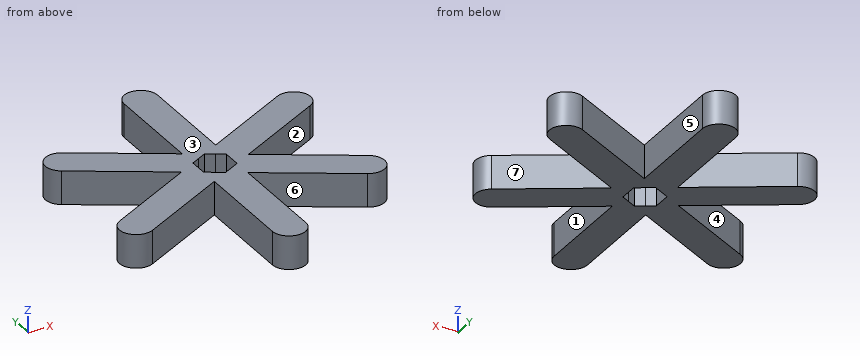
from build123d import *

# Parameters (mm, degrees)
F1_DEPTH = 12.7


with BuildPart() as f1:
    # F0 (on Top) → F1 (new body)
    with BuildSketch(Plane.XY):
        Polygon((-6.35, -3.6661742094), (-6.35, 0), (-6.35, 3.6661742094), (-12.7, 0), align=None)
        Polygon((0, -7.3323484187), (-3.175, -5.499261314), (-6.35, -3.6661742094), (-6.35, -10.9985226281), align=None)
        Polygon((6.35, 3.6661742094), (6.35, 0), (6.35, -3.6661742094), (12.7, 0), align=None)
        with BuildLine():
            Line((-12.7, 0), (-6.35, 3.6661742094))
            Line((-6.35, 3.6661742094), (-6.35, 10.9985226281))
            Line((-6.35, 10.9985226281), (-40.8190905122, 30.899261314))
            ThreePointArc((-40.8190905122, 30.899261314), (-49.4933518263, 28.575), (-47.1690905122, 19.900738686))
            Line((-47.1690905122, 19.900738686), (-12.7, 0))
        make_face()
        Polygon((-6.35, 10.9985226281), (-6.35, 3.6661742094), (-3.175, 5.499261314), (0, 7.3323484187), align=None)
        with BuildLine():
            Line((-6.35, -10.9985226281), (-6.35, -3.6661742094))
            Line((-6.35, -3.6661742094), (-12.7, 0))
            Line((-12.7, 0), (-47.1690905122, -19.900738686))
            ThreePointArc((-47.1690905122, -19.900738686), (-49.4933518263, -28.575), (-40.8190905122, -30.899261314))
            Line((-40.8190905122, -30.899261314), (-6.35, -10.9985226281))
        make_face()
        Polygon((6.35, -3.6661742094), (3.175, -5.499261314), (0, -7.3323484187), (6.35, -10.9985226281), align=None)
        with BuildLine():
            Line((6.35, -10.9985226281), (0, -7.3323484187))
            Line((0, -7.3323484187), (-6.35, -10.9985226281))
            Line((-6.35, -10.9985226281), (-6.35, -50.8))
            ThreePointArc((-6.35, -50.8), (0, -57.15), (6.35, -50.8))
            Line((6.35, -50.8), (6.35, -10.9985226281))
        make_face()
        Polygon((3.175, 5.499261314), (6.35, 3.6661742094), (6.35, 10.9985226281), (0, 7.3323484187), align=None)
        with BuildLine():
            Line((6.35, 10.9985226281), (6.35, 3.6661742094))
            Line((6.35, 3.6661742094), (12.7, 0))
            Line((12.7, 0), (47.1690905122, 19.900738686))
            ThreePointArc((47.1690905122, 19.900738686), (49.4933518263, 28.575), (40.8190905122, 30.899261314))
            Line((40.8190905122, 30.899261314), (6.35, 10.9985226281))
        make_face()
        with BuildLine():
            Line((12.7, 0), (6.35, -3.6661742094))
            Line((6.35, -3.6661742094), (6.35, -10.9985226281))
            Line((6.35, -10.9985226281), (40.8190905122, -30.899261314))
            ThreePointArc((40.8190905122, -30.899261314), (49.4933518263, -28.575), (47.1690905122, -19.900738686))
            Line((47.1690905122, -19.900738686), (12.7, 0))
        make_face()
        with BuildLine():
            Line((-6.35, 50.8), (-6.35, 10.9985226281))
            Line((-6.35, 10.9985226281), (0, 7.3323484187))
            Line((0, 7.3323484187), (6.35, 10.9985226281))
            Line((6.35, 10.9985226281), (6.35, 50.8))
            ThreePointArc((6.35, 50.8), (0, 57.15), (-6.35, 50.8))
        make_face()
    extrude(amount=-F1_DEPTH)


solid = f1.part
Could you check a few things on this model? Use its own coordinates, in mm. Face numbers are marked on the shaded views. A direction names the side the tool comes from. Round coordinates to 2 decimals unless told otherwise and drop trailing zeros. Loops run counter-clockwise (first coordinate to the right, second up) from the corner with the lowest first, then second, coordinate; pieces in that order, holes last. Notation, with made-up numbers: (78, 68.5) - (111, 68.5) arc R29 cw to (111, 102.5) - close; hole circle Ø5 at (-11, 50.5). An arc over 180 degrees is marked (long way). Write item = value, one per line.
1) Imagine slicing it at B-B (z = -2.5). Please give me the cut outline in (x, y) (3 decimals).
Computed:
outline = (-47.169, -19.901) arc R6.35 ccw to (-40.819, -30.899) - (-6.35, -10.999) - (-6.35, -50.8) arc R6.35 ccw to (6.35, -50.8) - (6.35, -10.999) - (40.819, -30.899) arc R6.35 ccw to (47.169, -19.901) - (12.7, 0) - (47.169, 19.901) arc R6.35 ccw to (40.819, 30.899) - (6.35, 10.999) - (6.35, 50.8) arc R6.35 ccw to (-6.35, 50.8) - (-6.35, 10.999) - (-40.819, 30.899) arc R6.35 ccw to (-47.169, 19.901) - (-12.7, 0) - close; hole (-6.35, -3.666) - (0, -7.332) - (6.35, -3.666) - (6.35, 3.666) - (0, 7.332) - (-6.35, 3.666) - close
2) If we mould it in two halves opening along X, with no side actions, what happens to the marked faces 1, 2 and 3? For each: pulls with the +X half, pulls with the -X half, needs draft (parallel to the pull), parting line crosses it, or undercut.
Computed:
face_1 = undercut
face_2 = pulls with the +X half
face_3 = needs draft
3) On a 3-axis mill with a long thin cutter (end or side, diameter ignored), from which of +Z, -Z, +X, -X, +Y, -Y can I reach the whole of each face in a straight line? I mean the marked faces 4, 5, 6 and 7. Say none if no direction works.
Computed:
face_4 = +Z, -Z, -X
face_5 = +Z, -Z, +Y
face_6 = +Z, -Z, -Y
face_7 = +Z, -Z, +X
4) Imagine slicing it at C-C (y = -13). Please give me the cut outline in (x, z), and give its area (3 significant figures).
Computed:
outline = (-35.22, -12.7) - (-9.82, -12.7) - (-9.82, 0) - (-35.22, 0) - close; (-6.35, -12.7) - (6.35, -12.7) - (6.35, 0) - (-6.35, 0) - close; (9.82, -12.7) - (35.22, -12.7) - (35.22, 0) - (9.82, 0) - close
area = 806 mm2
5) I'm going to push flat-ended pins straight in: P1, Ø4, axis at y = 21, z = -3.5, coming from the +X side; P2, Ø2, axis at y = 0, z = -4, coming from the -X side. Where does each tip first touch, or does it pass through?
Computed:
P1 = 49.87
P2 = -14.43
6) Imagine slicing it at A-A (x = 14). Please give me the cut outline in (y, z), and give its area (3 significant figures).
Computed:
outline = (-15.42, -12.7) - (-0.75, -12.7) - (-0.75, 0) - (-15.42, 0) - close; (0.75, -12.7) - (15.42, -12.7) - (15.42, 0) - (0.75, 0) - close
area = 372 mm2
7) I need wall thicknesses on line 1 along X through (y, z) = (-25.5, -5.25); line 2 along X through (y, z) = (-29, -11.75) (3 decimals); line 3 along X through (y, z) = (-44, -1). Which ranges of each line are inside material? Lowest first, please. Write a range as from..to.
Computed:
line_1 = -50.34..-31.47, -6.35..6.35, 31.47..50.34
line_2 = -49.225..-37.529, -6.35..6.35, 37.529..49.225
line_3 = -6.35..6.35
8) Imagine slicing it at D-D (y = -25.4). Please give me the cut outline in (x, z), and give its area (3 significant figures).
Computed:
outline = (-50.34, -12.7) - (-31.29, -12.7) - (-31.29, 0) - (-50.34, 0) - close; (-6.35, -12.7) - (6.35, -12.7) - (6.35, 0) - (-6.35, 0) - close; (31.29, -12.7) - (50.34, -12.7) - (50.34, 0) - (31.29, 0) - close
area = 645 mm2
